Input: part model. Units: mm. Frame: model coordinates. Face numbers are marked on the shaded views. A direction names the side the tool comes from. Coordinates: 2 decimals unless noted, no trailing zeros. Order: outer loops, then holes, each group sorted by start corner. A loop starts at its lowest first (then second) coordinate and runs counter-clockwise, first axis right, second up.
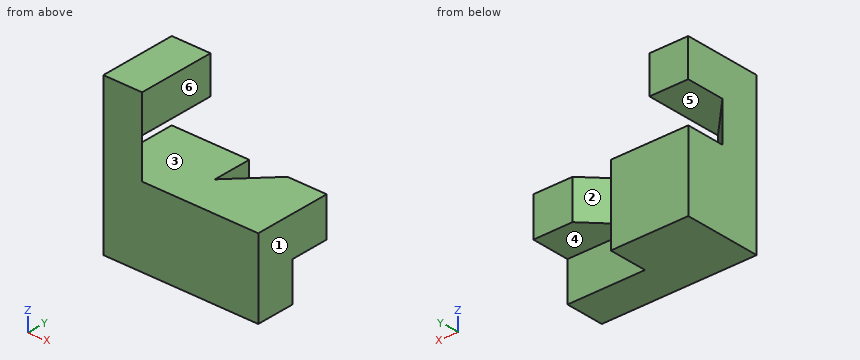
from build123d import *

# Parameters (mm, degrees)
F0_W      = 15.748
F0_H      = 15.748
F1_DEPTH  = 16.002
F3_DEPTH  = 8.128
F5_DEPTH  = 7.62
F6_W      = 7.874
F6_H      = 16.002
F7_DEPTH  = 15.748
F8_W      = 7.971476
F8_H      = 8.001
F9_DEPTH  = 7.874
F11_DEPTH = 8.001


with BuildPart() as f1:
    # F0 (on Top) → F1 (new body)
    with BuildSketch(Plane.XY):
        Rectangle(F0_W, F0_H)
    extrude(amount=F1_DEPTH)

    # F2 (on face) → F3 (join)
    with BuildSketch(Plane.XY.offset(16.002)):
        Polygon((0, -7.874), (-7.874, 0), (-7.874, -7.874), align=None)
    extrude(amount=F3_DEPTH)

    # F4 (on face) → F5 (join)
    with BuildSketch(Plane.XY.offset(24.13)):
        Polygon((-7.874, 0), (0, -7.874), (0, 7.889553), (-7.874, 7.889553), align=None)
        Polygon((-7.874, 0), (-7.874, -7.874), (0, -7.874), align=None)
    extrude(amount=F5_DEPTH)

    # F6 (on face) → F7 (join)
    with BuildSketch(Plane.YZ.offset(7.874)):
        with Locations((-3.937, 8.001)):
            Rectangle(F6_W, F6_H)
    extrude(amount=F7_DEPTH)

    # F8 (on face) → F9 (join, through all)
    with BuildSketch(Plane(origin=(0, 0, 0), x_dir=(-1, 0, 0), z_dir=(0, 1, 0))):
        with Locations((-19.636262, 12.0015)):
            Rectangle(F8_W, F8_H)
    extrude(amount=F9_DEPTH)

    # F10 (on face) → F11 (join, through all)
    with BuildSketch(Plane(origin=(0, 0, 8.001), x_dir=(1, 0, 0), z_dir=(0, 0, -1))):
        Polygon((7.865508, 0.029401), (15.650524, -7.874), (15.650524, 0), align=None)
    extrude(amount=-F11_DEPTH)


solid = f1.part
Item 1: Pin query (flat end, axial travel): pin 1 Ø4.5 at (x, y) = (9, 0.5) entering from +Z; pin 2 Ø4.5 at (x, z) = (19.5, 9) entering from +Y; pin 3 Ø4 at (y, z) = (2.5, 29) entering from +X. Return the tip coordinate at first contact, or that it passes through.
Response values:
pin 1: stops at z = 16
pin 2: stops at y = 7.87
pin 3: stops at x = 0
Item 2: Cut plane C-C on x = 22. Return loops of the section in (y, z).
Response values:
outline: (-7.87, 0) - (0, 0) - (0, 8) - (7.87, 8) - (7.87, 16) - (-7.87, 16) - close
Item 3: Draft query along X for the marked faces 1, 2 and 3. Return one class per face: pulls with the +X half, pulls with the -X half, needs draft (parallel to the pull), parting line crosses it, or undercut.
Response values:
face 1: pulls with the +X half
face 2: undercut
face 3: needs draft
Item 4: Cut plane D-D on y = 6.5. Return loops of the section in (x, z), then the cut area to 3 significant figures.
Response values:
outline: (-7.87, 0) - (7.87, 0) - (7.87, 16) - (-7.87, 16) - close; (-7.87, 24.13) - (0, 24.13) - (0, 31.75) - (-7.87, 31.75) - close; (14.3, 8) - (23.62, 8) - (23.62, 16) - (14.3, 16) - close
area: 387 mm2
Item 5: Cut plane A-A on y = 4.25. Return loops of the section in (x, z).
Response values:
outline: (-7.87, 0) - (7.87, 0) - (7.87, 16) - (-7.87, 16) - close; (-7.87, 24.13) - (0, 24.13) - (0, 31.75) - (-7.87, 31.75) - close; (12.08, 8) - (23.62, 8) - (23.62, 16) - (12.08, 16) - close
Item 6: Ray query, probe 1 along Z at (x, y) = (-5, 3.5); probe 2 along Y at (x, z) = (15.5, 1); probe 3 along Y at (x, z) = (21, 8.5). Return the intervals inside material, ascending.
Response values:
probe 1: z = 0 to 16, 24.13 to 31.75
probe 2: y = -7.87 to 0
probe 3: y = -7.87 to 7.87
Item 7: Access query for the marked faces 4, 5 and 6. Directions: +Z, -Z, +X, -X, +Y, -Y. A direction counts if a zero-diameter tool reaches every point of the face in a straight line with its end or side. Return the directions, or none.
Response values:
face 4: -Z, +X, +Y
face 5: +X, +Y
face 6: +Z, +X, +Y, -Y
